The model under review builds one solid part; all positions refer to its coordinate system, in mm. A direction names the side the tool comes from. Round coordinates to 2 decimals unless told otherwise and drop trailing zeros. Write each loop counter-clockwise with the first axis right and the second up, starting at its lowest first coordinate (ties: lowest second). Pieces come first, ordered by that corner, then holes. Notation, with made-up numbers: M -39.75,-7 L 10.25,-7 A29 ccw 10.25,14 Z; hole C 37,71.25 d2. An arc over 180 degrees is marked long. Write item = value, one per line. Start each with the question number.
Item 1: To check wall thickness, follow line 1 along X through (y, z) = (75, 40.5); line 2 along Z through (x, y) = (-99.5, 48); line 3 along Y through (x, z) = (0, 85). State the ranges of each line that lie inside material, in increasing order.
Item 2: Take a section at A-A, the plane y = -165.5. Give the boundary of the cut face in (x, z).
Item 3: The part is to be moulded in two halves that separate along X. For faces 6 (the flat face through (-2, 190.5, 44)), 7 (the flat face through (142, -3, 44)), 8 (the flat face through (-1, 1, 75)), say which applies: +X half, -X half, draft (parallel to the pull), parting line (faces both ways), or undercut.
Item 4: Tool access review of faces 1 (the cylindrical face through (21.77, 34.15, 82.6)), 2 (the cylindrical face through (-10.95, -49.3, 72.6)), 3 (the flat face through (-142, -3, 44)), 4 (the flat face through (-2, 45, 90)), 5 (the flat face through (-2, -2, 10)): name each direction out of +Z, -Z, +X, -X, +Y, -Y from which nothing blocks a thin tool from reaching the whole face with its end or side.
Item 5: Take a section at B-B, the plane x = -54.5. Give the boundary of the cut face in (y, z).
Item 6: For pin 1 Ø3 at (x, z) = (61, 73) entering from -Y, flat-tipped, find the tip position at first contact; note if it passes through.
Item 7: Take a section at C-C, the plane z = 29.5. Give the boundary of the cut face in (x, y), plus the area to 3 significant figures.
Item 8: Take a section at D-D, the plane y = 0. Give the boundary of the cut face in (x, z), plus the area to 3 significant figures.
from build123d import *

# Parameters (mm, degrees)
SKETCH1_W           = 284
SKETCH1_H           = 381
BOSS_EXTRUDE1_DEPTH = 60
SKETCH3_W           = 284
SKETCH3_H           = 381
BOSS_EXTRUDE2_DEPTH = 30
SKETCH4_R           = 40.5
CUT_EXTRUDE1_DEPTH  = 15
SHELL1_T            = -10
FILLET1_R           = 2


with BuildPart() as part:
    # Sketch1 → Boss-Extrude1 (new body)
    with BuildSketch(Plane.XY):
        Rectangle(SKETCH1_W, SKETCH1_H)
    extrude(amount=BOSS_EXTRUDE1_DEPTH)

    # Sketch3 → Boss-Extrude2 (add)
    with BuildSketch(Plane.XY.offset(60)):
        Rectangle(SKETCH3_W, SKETCH3_H)
    extrude(amount=BOSS_EXTRUDE2_DEPTH)

    # Sketch4 → Cut-Extrude1 (cut)
    with BuildSketch(Plane.XY.offset(90)):
        Circle(SKETCH4_R)
    extrude(amount=-CUT_EXTRUDE1_DEPTH, mode=Mode.SUBTRACT)

    # Shell1
    shell1_openings = [part.faces().sort_by_distance(p)[0] for p in [
        (0, -190.5, 45),
    ]]
    offset(amount=SHELL1_T, openings=shell1_openings, kind=Kind.INTERSECTION)

    # Fillet1
    fillet1_edges = [part.edges().sort_by_distance(p)[0] for p in [
        (142, -190.5, 45),
        (-142, -190.5, 45),
        (-142, 190.5, 45),
        (142, 190.5, 45),
    ]]
    fillet(fillet1_edges, radius=FILLET1_R)


solid = part.part
Response values:
q1.line_1 = -142 to -132, 132 to 142
q1.line_2 = 0 to 10, 80 to 90
q1.line_3 = -190.5 to -40.5, 40.5 to 190.5
q2.outline = M -142,0 L 142,0 L 142,90 L -142,90 Z; hole M -132,10 L 132,10 L 132,80 L -132,80 Z
q3.face_6 = draft
q3.face_7 = +X half
q3.face_8 = undercut
q4.face_1 = +Z
q4.face_2 = none
q4.face_3 = +Z, -Z, -X, +Y, -Y
q4.face_4 = +Z, +X, -X, +Y, -Y
q4.face_5 = -Y
q5.outline = M -190.5,0 L 190.5,0 L 190.5,90 L -190.5,90 L -190.5,80 L 180.5,80 L 180.5,10 L -190.5,10 Z
q6.pin_1 = 180.5
q7.outline = M -142,-188.5 A2 ccw -140,-190.5 L -132,-190.5 L -132,180.5 L 132,180.5 L 132,-190.5 L 140,-190.5 A2 ccw 142,-188.5 L 142,188.5 A2 ccw 140,190.5 L -140,190.5 A2 ccw -142,188.5 Z
q7.area = 10,300 mm2
q8.outline = M -142,0 L 142,0 L 142,90 L 40.5,90 L 40.5,75 L -40.5,75 L -40.5,90 L -142,90 Z; hole M -132,10 L 132,10 L 132,80 L 50.5,80 L 50.5,65 L -50.5,65 L -50.5,80 L -132,80 Z
q8.area = 7,380 mm2
